Here's how the part is built. I have some questions about the finished solid (model axes, mm). Round coordinates to 2 decimals unless told otherwise and drop trailing zeros. Write each loop counter-clockwise with the first axis right and the second up, starting at its lowest first coordinate (ties: lowest second). Pieces come first, ordered by that corner, then holes. Notation, with made-up numbers: (56, 81) - (62, 81) arc R27 cw to (62, 101) - close; hole circle Ø3 at (61.25, -26). An arc over 180 degrees is marked (long way). One line per question, with ' | ' between items. Start each with the question number.
(1) Imagine slicing it at A-A (z = -251.5). Write out the boundary of the cut face in (x, y).
(2) If I drill on L1, parallel to X at y = 3.6, z = -290; L2, parallel to Z at x = 290, y = 2.5; L3, parallel to Z at x = 242, y = 16.75, over which ranges is the centre line in solid material (lowest first)?
(3) Imagine slicing it at D-D (x = 273.5). Write out the boundary of the cut face in (y, z), plus the area to 3 significant figures.
(4) Imagine slicing it at C-C (x = 242.5). Write out the boundary of the cut face in (y, z), plus the area to 3 significant figures.
(5) Will these pins go through, and if not, where does the flat tip stop? pin 1 (5 mm diameter, centred on y = 22.5, z = -169, fed in from +X); pin 2 (1 mm diameter, centred on x = 126, y = 16, fed in from +Z); pin 3 (7.5 mm diameter, centred on y = 17.5, z = -193.5, fed in from -X).
(6) Imagine slicing it at B-B (y = 16.5). Write out the boundary of the cut face in (x, z), plus the area to 4 significant figures.
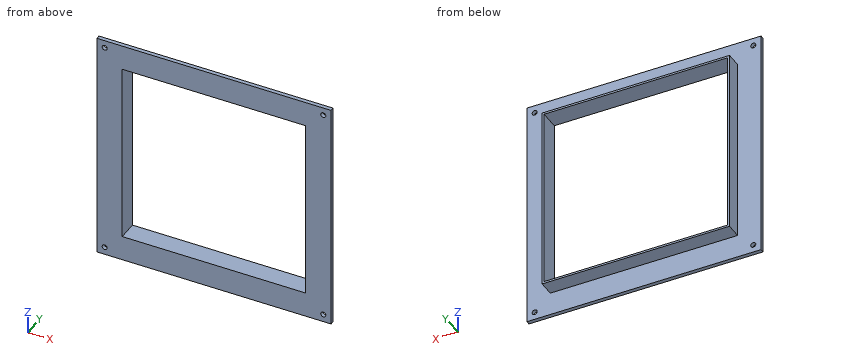
from build123d import *

# Parameters (mm, degrees)
BOSS_EXTRUDE1_DEPTH = 5
SKETCH4_W           = 240
SKETCH4_H           = 240
SKETCH4_W_2         = 230.5
SKETCH4_H_2         = 230.5
BOSS_EXTRUDE2_DEPTH = 20
SKETCH6_R           = 3.25
CUT_EXTRUDE1_DEPTH  = 20
SKETCH7_W           = 240
SKETCH7_H           = 240
CUT_EXTRUDE2_DEPTH  = 20
SKETCH8_W           = 240
SKETCH8_H           = 240
SKETCH8_W_2         = 235
SKETCH8_H_2         = 235
BOSS_EXTRUDE3_DEPTH = 20
SKETCH9_W           = 235
SKETCH9_H           = 235
CUT_EXTRUDE3_DEPTH  = 20


with BuildPart() as part:
    # Sketch3 → Boss-Extrude1 (new body)
    with BuildSketch(Plane(origin=(0, 0, 0), x_dir=(1, 0, 0), z_dir=(0, 1, 0))):
        Polygon((300, 300), (150, 150), (300, 0), align=None)
        Polygon((150, 150), (0, 0), (300, 0), align=None)
        Polygon((0, 300), (0, 0), (150, 150), align=None)
        Polygon((0, 300), (150, 150), (300, 300), align=None)
    extrude(amount=BOSS_EXTRUDE1_DEPTH)

    # Sketch4 → Boss-Extrude2 (add)
    with BuildSketch(Plane(origin=(0, 5, 0), x_dir=(1, 0, 0), z_dir=(0, 1, 0))):
        with Locations((150, 150)):
            Rectangle(SKETCH4_W, SKETCH4_H)
        with Locations((150, 150)):
            Rectangle(SKETCH4_W_2, SKETCH4_H_2, mode=Mode.SUBTRACT)
    extrude(amount=BOSS_EXTRUDE2_DEPTH)

    # Sketch6 → Cut-Extrude1 (cut)
    with BuildSketch(Plane(origin=(0, 5, 0), x_dir=(1, 0, 0), z_dir=(0, 1, 0))):
        with Locations(Location((10, 10, 0), (0, 0, 270))):
            Circle(SKETCH6_R)
        with Locations(Location((290, 10, 0), (0, 0, 270))):
            Circle(SKETCH6_R)
        with Locations(Location((290, 290, 0), (0, 0, 270))):
            Circle(SKETCH6_R)
        with Locations(Location((10, 290, 0), (0, 0, 270))):
            Circle(SKETCH6_R)
    extrude(amount=-CUT_EXTRUDE1_DEPTH, mode=Mode.SUBTRACT)

    # Sketch7 → Cut-Extrude2 (cut)
    with BuildSketch(Plane(origin=(0, 25, 0), x_dir=(1, 0, 0), z_dir=(0, 1, 0))):
        with Locations((150, 150)):
            Rectangle(SKETCH7_W, SKETCH7_H)
    extrude(amount=-CUT_EXTRUDE2_DEPTH, mode=Mode.SUBTRACT)

    # Sketch8 → Boss-Extrude3 (add)
    with BuildSketch(Plane(origin=(0, 5, 0), x_dir=(1, 0, 0), z_dir=(0, 1, 0))):
        with Locations((150, 150)):
            Rectangle(SKETCH8_W, SKETCH8_H)
        with Locations((150, 150)):
            Rectangle(SKETCH8_W_2, SKETCH8_H_2, mode=Mode.SUBTRACT)
    extrude(amount=BOSS_EXTRUDE3_DEPTH)

    # Sketch9 → Cut-Extrude3 (cut)
    with BuildSketch(Plane(origin=(0, 5, 0), x_dir=(1, 0, 0), z_dir=(0, 1, 0))):
        with Locations((150, 150)):
            Rectangle(SKETCH9_W, SKETCH9_H)
    extrude(amount=-CUT_EXTRUDE3_DEPTH, mode=Mode.SUBTRACT)


solid = part.part
Check sheet entries:
1) outline: (0, 0) - (32.5, 0) - (32.5, 25) - (30, 25) - (30, 5) - (0, 5) - close; (267.5, 0) - (300, 0) - (300, 5) - (270, 5) - (270, 25) - (267.5, 25) - close
2) L1: 0 to 6.75, 13.25 to 286.75, 293.25 to 300 | L2: -300 to -293.25, -286.75 to -13.25, -6.75 to 0 | L3: -270 to -267.5, -32.5 to -30
3) outline: (0, -300) - (5, -300) - (5, 0) - (0, 0) - close | area: 1,500 mm^2
4) outline: (0, -300) - (5, -300) - (5, -270) - (25, -270) - (25, -267.5) - (0, -267.5) - close; (0, -32.5) - (25, -32.5) - (25, -30) - (5, -30) - (5, 0) - (0, 0) - close | area: 425 mm^2
5) pin 1: x = 270 | pin 2: z = -30 | pin 3: x = 30
6) outline: (30, -270) - (270, -270) - (270, -30) - (30, -30) - close; hole (32.5, -267.5) - (267.5, -267.5) - (267.5, -32.5) - (32.5, -32.5) - close | area: 2,375 mm^2
